```python
from build123d import *

# Parameters (mm, degrees)
F0_R     = 15
F0_R_2   = 10
F1_DEPTH = 25
F2_DEPTH = 50
F3_R     = 5.08
F4_SIZE  = 3


with BuildPart() as f1:
    # F0 (on Front) → F1 (new body)
    with BuildSketch(Plane.XZ):
        with BuildLine():
            ThreePointArc((6.25, -29.3417364858), (23.3184476327, -18.8745860882), (30, 0))
            ThreePointArc((30, 0), (23.3184476327, 18.8745860882), (6.25, 29.3417364858))
            ThreePointArc((6.25, 29.3417364858), (-30, 0), (6.25, -29.3417364858))
        make_face()
        Circle(F0_R, mode=Mode.SUBTRACT)
        with BuildLine():
            ThreePointArc((6.25, 29.3417364858), (23.3184476327, 18.8745860882), (30, 0))
            ThreePointArc((30, 0), (23.3184476327, -18.8745860882), (6.25, -29.3417364858))
            Line((6.25, -29.3417364858), (63.6458333333, -17.11601295))
            ThreePointArc((63.6458333333, -17.11601295), (42.5, 0), (63.6458333333, 17.11601295))
            Line((63.6458333333, 17.11601295), (6.25, 29.3417364858))
        make_face()
        with BuildLine():
            ThreePointArc((77.5, 0), (73.6024277858, 11.0101752181), (63.6458333333, 17.11601295))
            ThreePointArc((63.6458333333, 17.11601295), (42.5, 0), (63.6458333333, -17.11601295))
            ThreePointArc((63.6458333333, -17.11601295), (73.6024277858, -11.0101752181), (77.5, 0))
        make_face()
        with Locations((60, 0)):
            Circle(F0_R_2, mode=Mode.SUBTRACT)
    extrude(amount=F1_DEPTH)

    # F0 (on Front) → F2 (join)
    with BuildSketch(Plane.XZ):
        with BuildLine():
            ThreePointArc((6.25, -29.3417364858), (23.3184476327, -18.8745860882), (30, 0))
            ThreePointArc((30, 0), (23.3184476327, 18.8745860882), (6.25, 29.3417364858))
            ThreePointArc((6.25, 29.3417364858), (-30, 0), (6.25, -29.3417364858))
        make_face()
        Circle(F0_R, mode=Mode.SUBTRACT)
    extrude(amount=F2_DEPTH)

    # F3
    f3_edges = [f1.edges().sort_by_distance(p)[0] for p in [
        (34.947917, 0, -23.228875),
        (-6.25, -50, 29.341736),
    ]]
    fillet(f3_edges, radius=F3_R)

    # F4
    f4_edges = [f1.edges().sort_by_distance(p)[0] for p in [
        (-15, -50, 0),
        (-5.191667, -50, 24.373202),
        (50, -25, 0),
    ]]
    chamfer(f4_edges, length=F4_SIZE)


solid = f1.part
```
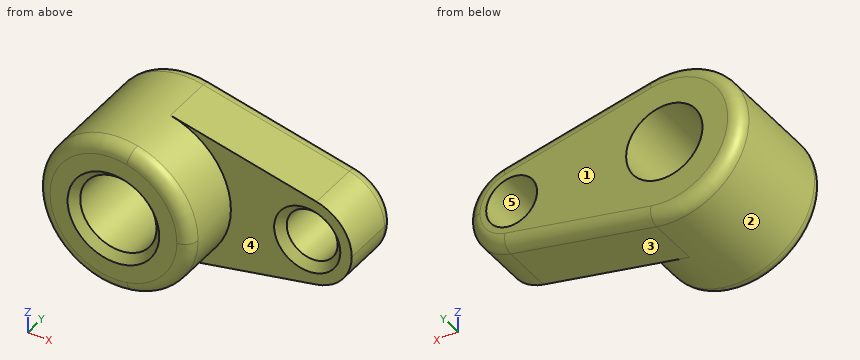
The listing builds one solid part. Answer for the finished solid, in the listing's coordinates (mm). Face numbers are marked on the shaded views. A direction names the side the tool comes from. Give positions to 0.01 mm unless a question says otherwise; leave off trailing zeros. Put each result on its own line as item: value. Start each with the question number.
Item 1: The part is cut by section A-A, the plane z = -3. State how many separate pieces and enclosed holes the cut face has, and give its area (3 significant figures).
Item 2: Flat-ended cylindrical pins translate along their axes: P1, Ø1, axis at x = -13.5, y = -42, coming from the +Z side; P2, Ø2, axis at y = -38, z = 5.5, coming from the -X side; P3, Ø6, axis at x = 27, y = -23.5, coming from the -Z side. Find the tip coordinate at first contact, or state that the pin passes through.
Item 3: Find the intervals of material crossed by line 1 along Z through (x, y) = (0, -13.5); line 2 along X through (y, z) = (-4, 5.5); line 3 along Y through (x, z) = (52.5, 13.5), in increasing order.
Item 4: Which of the six approach directions +Z, -Z, +X, -X, +Y, -Y give full straight-line access (tool end or side, diameter ignored) to the marked faces 1 and 2?
Item 5: For a pull along Z with two mould halves and no side action, classify the marked faces 3, 4 and 5 as +Z half, -Z half, draft (parallel to the pull), parting line (faces both ways), or undercut.
Answer key:
1. separate pieces: 3
1. enclosed holes: 0
1. area: 2,180 mm²
2. P1: stops at z = 27.04
2. P2: stops at x = -29.66
2. P3: stops at z = -25.56
3. line 1: z = -30 to -15, 15 to 30
3. line 2: x = -29.37 to -13.96, 13.96 to 51.65, 68.35 to 76.49
3. line 3: y = -25 to 0
4. face 1: +Z, -Z, +X, -X, +Y
4. face 2: -Y
5. face 3: -Z half
5. face 4: draft
5. face 5: undercut
